Can you work these out from the model? Positions are in its coordinate system, mm. Face numbers are marked on the shaded views. Give positions to 0.01 mm unless a question says otherwise; leave off trailing zeros. Loops run counter-clockwise (first coordinate to the right, second up) from the corner with the lowest first, then second, coordinate; pieces in that order, holes last.
from build123d import *

# Parameters (mm, degrees)
SKETCH1_R      = 74
EXTRUDE1_DEPTH = 30
SKETCH2_R      = 64
EXTRUDE2_DEPTH = 300
SHELL1_T       = -10
FILLET2_R      = 5
CHAMFER2_SIZE  = 2
SKETCH3_R      = 20
EXTRUDE3_DEPTH = 347.196476007
CHAMFER3_SIZE  = 2


with BuildPart() as part:
    # Sketch1 → Extrude1 (new body)
    with BuildSketch(Plane.XY):
        Circle(SKETCH1_R)
    extrude(amount=EXTRUDE1_DEPTH)

    # Sketch2 → Extrude2 (add)
    with BuildSketch(Plane.XY.offset(30)):
        Circle(SKETCH2_R)
    extrude(amount=EXTRUDE2_DEPTH)

    # Shell1
    shell1_openings = [part.faces().sort_by_distance(p)[0] for p in [
        (0, 0, 0),
    ]]
    offset(amount=SHELL1_T, openings=shell1_openings, kind=Kind.INTERSECTION)

    # Fillet2
    fillet2_edges = [part.edges().sort_by_distance(p)[0] for p in [
        (-64, 0, 30),
    ]]
    fillet(fillet2_edges, radius=FILLET2_R)

    # Chamfer2
    chamfer2_edges = [part.edges().sort_by_distance(p)[0] for p in [
        (-64, 0, 330),
    ]]
    chamfer(chamfer2_edges, length=CHAMFER2_SIZE)

    # Sketch3 → Extrude3 (cut, through all)
    with BuildSketch(Plane.XY.offset(330)):
        Circle(SKETCH3_R)
    extrude(amount=-EXTRUDE3_DEPTH, mode=Mode.SUBTRACT)

    # Chamfer3
    chamfer3_edges = [part.edges().sort_by_distance(p)[0] for p in [
        (-20, 0, 320),
        (-20, 0, 330),
    ]]
    chamfer(chamfer3_edges, length=CHAMFER3_SIZE)


solid = part.part
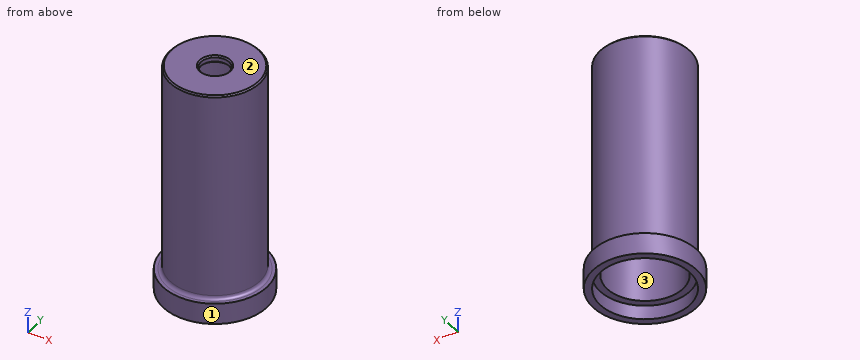
(1) Suppose I cut it at A-A on x = 0. List the corners of the cut face in (y, z) for me, plus the area to 3 significant figures.
Returned:
outline: (-74, 0) - (-64, 0) - (-64, 20) - (-54, 20) - (-54, 320) - (-22, 320) - (-20, 322) - (-20, 328) - (-22, 330) - (-62, 330) - (-64, 328) - (-64, 35) arc R5 cw to (-69, 30) - (-74, 30) - close; (20, 322) - (22, 320) - (54, 320) - (54, 20) - (64, 20) - (64, 0) - (74, 0) - (74, 30) - (69, 30) arc R5 cw to (64, 35) - (64, 328) - (62, 330) - (22, 330) - (20, 328) - close
area: 7,480 mm2
(2) Thinking about a two-plate mould opening in Y: for the marked faces 1, 2 and 3, which applies, pulls with the +Y half, pulls with the -Y half, needs draft (parallel to the pull), parting line crosses it, or undercut?
Returned:
face 1: parting line crosses it
face 2: needs draft
face 3: undercut
(3) Will these pins go through, and if not, where does the flat tip stop? P1, Ø12, axis at x = 14, z = 291, coming from the -Y side; P2, Ø3, axis at y = 33.5, z = 248, coming from the +X side; P3, Ø12, axis at x = -17.5, z = 235.5, coming from the +Y side.
Returned:
P1: stops at y = -63.5
P2: stops at x = 55.43
P3: stops at y = 62.96
(4) Suppose I cut it at C-C on z = 276. List the corners of the cut face in (x, y) for me.
Returned:
outline: circle Ø128 at (0, 0); hole circle Ø108 at (0, 0)
(5) Please list where these lines run through material, in increasing order: probe 1 along Y at (x, z) = (0, 325.7); probe 2 along Y at (x, z) = (1.5, 113.5); probe 3 along Z at (x, y) = (-15.5, 26.5).
Returned:
probe 1: y = -64 to -20, 20 to 64
probe 2: y = -63.98 to -53.98, 53.98 to 63.98
probe 3: z = 320 to 330
